```python
from build123d import *

# Parameters (mm, degrees)
SKETCH_1_R               = 15
EXTRUDE_1_DEPTH          = 65
SKETCH_2_R               = 17.5
EXTRUDE_4_DEPTH          = 15
CUT_EXTRUDE_1_DEPTH      = 89.069574902
CUT_EXTRUDE_1_DEPTH_BACK = 89.069574902
SKETCH_3_R               = 11


with BuildPart() as part:
    # 스케치1 → 보스-돌출1 (new, symmetric)
    with BuildSketch(Plane(origin=(0, 0, 0), x_dir=(1, 0, 0), z_dir=(0, 1, 0))):
        with Locations(Location((0, 0, 0), (0, 0, 270))):
            Circle(SKETCH_1_R)
    extrude(amount=EXTRUDE_1_DEPTH, both=True)

    # 스케치2 → 보스-돌출4 (add, symmetric)
    with BuildSketch(Plane.XY):
        with Locations((0, 67.5)):
            Circle(SKETCH_2_R)
    extrude(amount=EXTRUDE_4_DEPTH, both=True)

    # 스케치3 → 컷-돌출1 (cut, two sides: drawn at the far end of the back side and taken through both)
    with BuildSketch(Plane.XY.offset(-CUT_EXTRUDE_1_DEPTH_BACK)):
        with Locations((0, 67.5)):
            Circle(SKETCH_3_R)
    extrude(amount=CUT_EXTRUDE_1_DEPTH + CUT_EXTRUDE_1_DEPTH_BACK, mode=Mode.SUBTRACT)


solid = part.part
```
Could you check a few things on this model? Use its own coordinates, in mm. Coordinates: 2 decimals unless noted, no trailing zeros. Order: outer loops, then holes, each group sorted by start corner. A loop starts at its lowest first (then second) coordinate and runs counter-clockwise, first axis right, second up. Notation, with made-up numbers: M 32.5,56 L 58.5,56 A8 cw 58.5,61 Z; hole C 19,-12.5 d11. An arc over 180 degrees is marked long. Use a Markdown table: item, result. Add a question column.
Q1. I want a section at D-D on x = 6. List the corners of the cut face in (y, z) for me, then the cut area to 3 significant figures.
Q2. We'd pull the mould along Y, two halves only. Please class faces 1 (the cylindrical face through (-1.432, 78.406, -0.21)), 2 (the flat face through (0, -65, 0)), 3 (the cylindrical face through (0.66, -2.392, -14.985)): pulls with the +Y half, pulls with the -Y half, needs draft (parallel to the pull), parting line crosses it, or undercut.
Q3. If I drill on L1, parallel to X at y = 67.5, z = -8.5; L2, parallel to X at y = 73, z = -12.5; L3, parallel to Y at x = -4.5, z = 10, over which ranges is the centre line in solid material (lowest first)?
Q4. I'm going to push flat-ended pins straight in: pin 1 (2 mm diameter, centred on x = -2, y = -29.5, fed in from +Z); pin 2 (2 mm diameter, centred on x = 5.5, z = -11.5, fed in from +Y); pin 3 (3 mm diameter, centred on x = 6, y = 28.5, fed in from -Z); pin 4 (13 mm diameter, centred on x = 0, y = 67.5, fed in from -Z). Where does each tip first touch, or does it pass through?
Q5. I want a section at A-A on y = 67.5. List the corners of the cut face in (x, z) for me.
Q6. I want a section at B-B on x = -7.5. List the corners of the cut face in (y, z) for me, then the cut area to 3 significant figures.
Checked values:
| question | item | result |
|---|---|---|
| 1 | outline | M -65,-13.75 L 51.06,-13.75 L 51.06,-15 L 58.28,-15 L 58.28,15 L 51.06,15 L 51.06,13.75 L -65,13.75 Z; M 76.72,-15 L 83.94,-15 L 83.94,15 L 76.72,15 Z |
| 1 | area | 3,620 mm² |
| 2 | face 1 | undercut |
| 2 | face 2 | pulls with the -Y half |
| 2 | face 3 | needs draft |
| 3 | L1 | -17.5 to -11, 11 to 17.5 |
| 3 | L2 | -16.61 to -9.53, 9.53 to 16.61 |
| 3 | L3 | -65 to 57.46, 77.54 to 84.41 |
| 4 | pin 1 | z = 14.97 |
| 4 | pin 2 | y = 84.41 |
| 4 | pin 3 | z = -14.31 |
| 4 | pin 4 | through |
| 5 | outline | M -17.5,-15 L -11,-15 L -11,15 L -17.5,15 Z; M 11,-15 L 17.5,-15 L 17.5,15 L 11,15 Z |
| 6 | outline | M -65,-12.99 L 51.69,-12.99 L 51.69,-15 L 59.45,-15 L 59.45,15 L 51.69,15 L 51.69,12.99 L -65,12.99 Z; M 75.55,-15 L 83.31,-15 L 83.31,15 L 75.55,15 Z |
| 6 | area | 3,500 mm² |
